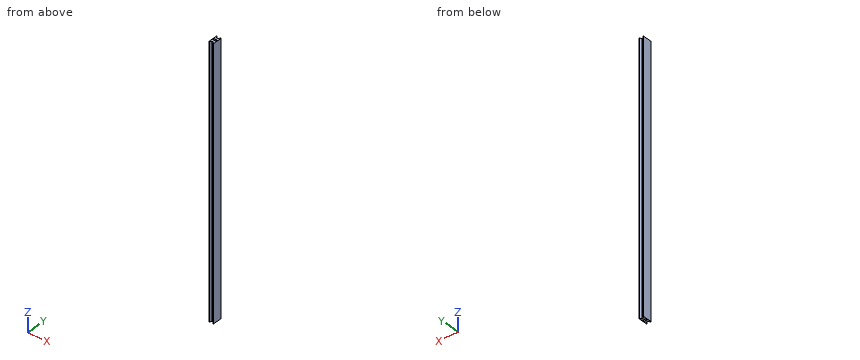
Autodesk Inventor part; units mm, degrees
ref_plane "YZ Plane" through (0, 0, 0) normal (1, 0, 0) x (0, 1, 0)
ref_plane "XZ Plane" through (0, 0, 0) normal (0, 1, 0) x (-1, 0, 0)
ref_plane "XY Plane" through (0, 0, 0) normal (0, 0, 1) x (1, 0, 0)
sketch "Sketch1" plane through (0, 0, 0) normal (0, 0, 1) x (1, 0, 0)
  line L0 (0, 0) -> (50, 0)
  line L1 (50, 0) -> (50, 100)
  line L2 (50, 100) -> (0, 100)
  line L3 (0, 100) -> (0, 0)
  dimension "d0" = 50
  dimension "d1" = 100
extrude "Extrusion1" add sketch "Sketch1" along normal blind 2900
sketch "Sketch2" plane through (0, 0, 2900) normal (0, 0, 1) x (1, 0, 0)
  line L0 (0, 0) -> (50, 0)
  line L1 (50, 0) -> (50, 100)
  line L2 (50, 100) -> (0, 100)
  line L3 (0, 100) -> (0, 0)
  line L4 (16.6667, 80) -> (33.3333, 80)
  line L5 (16.6667, 80) -> (43.3333, 80) construction
  line L6 (16.6667, 80) -> (5.1197, 100)
  line L7 (50, 100) -> (0, 100)
  line L8 (16.6667, 80) -> (39.7607, 80) construction
  line L9 (33.3333, 80) -> (44.8803, 100)
  line L10 (33.3333, 80) -> (56.4273, 80) construction
  line L11 (44.8803, 100) -> (5.1197, 100)
  line L12 (0, 50) -> (50, 50)
  line L13 (50, 0) -> (50, 100)
  line L14 (16.6667, 20) -> (33.3333, 20)
  line L15 (16.6667, 20) -> (5.1197, 0)
  line L16 (33.3333, 20) -> (44.8803, 0)
  line L17 (44.8803, 0) -> (5.1197, 0)
  dimension "d4" = 50
  dimension "d5" = 16.6667
  dimension "d6" = 100
  dimension "d7" = 20
  dimension "d8" = 16.6667
  dimension "d11" = 120
  dimension "d12" = 60
  dimension "d13" = 50
extrude "Extrusion2" cut sketch "Sketch2" against normal up to next contours L15 L14 L16 L0 | L2 L9 L4 L6
sketch "Sketch3" plane through (0, 0, 2900) normal (0, 0, 1) x (1, 0, 0)
  line L0 (33.3333, 80) -> (16.6667, 80)
  line L1 (16.6667, 60) -> (33.3333, 60)
  line L2 (0, 100) -> (0, 0)
  line L3 (16.6667, 20) -> (33.3333, 20)
  line L4 (50, 100) -> (44.8803, 100)
  line L5 (16.6667, 40) -> (33.3333, 40)
  line L6 (5.1197, 56.6667) -> (5.1197, 43.3333)
  line L7 (25, 80) -> (25, 20)
  line L8 (16.6667, 60) -> (5.1197, 56.6667)
  line L9 (16.6667, 40) -> (5.1197, 43.3333)
  line L10 (44.8803, 56.6667) -> (44.8803, 43.3333)
  line L11 (33.3333, 60) -> (44.8803, 56.6667)
  line L12 (33.3333, 40) -> (44.8803, 43.3333)
  dimension "d16" = 16.6667
  dimension "d17" = 16.6667
  dimension "d18" = 16.6667
  dimension "d19" = 16.6667
  dimension "d20" = 20
  dimension "d21" = 20
  dimension "d22" = 100
  dimension "d23" = 16.6667
  dimension "d25" = 40
  dimension "d26" = 16.6667
  dimension "d27" = 13.3333
  dimension "d28" = 3.3333
extrude "Extrusion3" cut sketch "Sketch3" against normal blind 2900
equation "\"d1\" = 2 * d0"
equation "\"d5\" = 0.333333 * d4"
equation "\"d7\" = 0.2 * d6"
equation "\"d8\" = -0.5 * d5 + 0.5 * d4"
equation "\"d13\" = 0.5 * d6"
equation "\"d17\" = d16"
equation "\"d19\" = d18"
equation "\"d21\" = 0.5 * d22 - 1.5 * d20"
equation "\"d23\" = d24"
equation "\"d25\" = -0.5 * d20 + 0.5 * d22"
equation "\"d26\" = d16"
equation "\"d27\" = 0.666667 * d21"
equation "\"d28\" = -0.5 * d27 + 0.5 * d21"
properties part number "wheelRoad"
The listing builds one solid part. Answer for the finished solid, in the listing's coordinates (mm). Give positions to 0.01 mm unless a question says otherwise; leave off trailing zeros. Write each loop counter-clockwise with the first axis right and the second up, starting at its lowest first coordinate (ties: lowest second). Pieces come first, ordered by that corner, then holes.
Item 1: Flat-ended cylindrical pins translate along their axes: P1, Ø10, axis at x = 41.5, y = 65, coming from the -Z side; P2, Ø18.5, axis at x = 27.5, z = 1559.5, coming from the +Y side; P3, Ø4, axis at x = 7.5, z = 1182.5, coming from the -Y side; P4, Ø13.5, axis at x = 27.5, z = 817, coming from the -Y side. Find the tip coordinate at first contact, or state that the pin passes through.
Item 2: Find the intervals of material crossed by line 1 along X through (y, z) = (50, 2391.5); line 2 along Y through (x, z) = (31, 980.5); line 3 along X through (y, z) = (89, 867.5), in increasing order.
Item 3: Section A-A, the plane z = 2109 is taken. Write down the section's boundary in (x, y).
Completed:
1. P1: stops at z = 0
1. P2: stops at y = 85.92
1. P3: stops at y = 0.66
1. P4: stops at y = 18.41
2. line 1: x = 0 to 5.12, 44.88 to 50
2. line 2: y = 20 to 40, 60 to 80
2. line 3: x = 0 to 11.47, 38.53 to 50
3. outline: (0, 0) - (5.12, 0) - (16.67, 20) - (33.33, 20) - (44.88, 0) - (50, 0) - (50, 100) - (44.88, 100) - (33.33, 80) - (16.67, 80) - (5.12, 100) - (0, 100) - close; hole (5.12, 43.33) - (16.67, 40) - (33.33, 40) - (44.88, 43.33) - (44.88, 56.67) - (33.33, 60) - (16.67, 60) - (5.12, 56.67) - close
